Geometry: final body of the model. Coordinates: model frame, mm. A direction names the side the tool comes from. Give positions to 0.01 mm unless a question says otherwise; leave off trailing zeros. Order: outer loops, then holes, each group sorted by start corner. A loop starts at its lowest first (then second) coordinate and runs counter-clockwise, first axis right, second up. Notation, with made-up numbers: (52, 30.5) -> (70, 30.5) arc R6 cw to (70, 37.5) -> close; hole circle Ø8 at (57.5, 86). An arc over 180 degrees is marked (long way). One line per question, with ' | ' between items. Start each with the question number.
(1) Section D-D (x = 67.5). Return loops of the section in (y, z), then the cut area to 3 significant figures.
(2) Mould query, pull axis Y, two halves, no side actions, for faces 5 (the face through (45.44, 40.45, -2.54)), 6 (the face through (-3, 1, -2)), 7 (the face through (2, 3.05, -2)), 8 (the face through (35, 124, -2)). Classes: +Y half, -Y half, draft (parallel to the pull), parting line (faces both ways), or undercut.
(3) Ray query, L1, parallel to Y at x = 28, z = -59.5; L2, parallel to Y at x = 45, z = -3.2; L3, parallel to Z at x = 51, y = 67. Return the intervals inside material, ascending.
(4) First-contact query: pin 1 Ø12 at (y, z) = (80, -24) entering from -X; pin 2 Ø5.5 at (y, z) = (116.5, -3) entering from -X; pin 3 Ø4.5 at (x, z) = (-2, -3.5) entering from -Y. Flat tips, straight axial feed; report the tip coordinate or a pass-through.
(5) Set-up query: faces 1 (the face through (18, 149, -28)), 2 (the face through (-3, -1, -2)), 3 (the face through (50, 75.95, -32)), 4 (the face through (7, -3.05, -2)). Return all of +Z, -Z, +X, -X, +Y, -Y with unobstructed straight access to the full face (end or side cutting, diameter ignored); none if empty.
(6) Section C-C (y = 113). Return loops of the section in (x, z).
(7) Section A-A (z = -45). Return loops of the section in (x, y).
(8) Section B-B (x = 17.5). Return loops of the section in (y, z).
```python
from build123d import *

# Parameters (mm, degrees)
BOSS_EXTRUDE1_DEPTH = 5
BOSS_EXTRUDE2_DEPTH = 80
SKETCH4_W           = 4
SKETCH4_H           = 2
CUT_EXTRUDE1_DEPTH  = 73.715728753
SKETCH5_W           = 67.715728753
SKETCH5_H           = 50
CUT_EXTRUDE2_DEPTH  = 81
CUT_EXTRUDE3_DEPTH  = 65
SKETCH7_W           = 80
SKETCH7_H           = 5
BOSS_EXTRUDE3_DEPTH = 10.5
BOSS_EXTRUDE4_DEPTH = 80
FILLET1_R           = 2
FILLET2_R           = 10
CUT_EXTRUDE4_DEPTH  = 170.5
FILLET3_R           = 10
SKETCH10_R          = 3.4
CUT_EXTRUDE5_DEPTH  = 6


with BuildPart() as part:
    # Sketch2 → Boss-Extrude1 (new body)
    with BuildSketch(Plane.XY):
        Polygon((-5.152414984, 3.618325464), (-5.152414984, -3.618325464), (-1.641080211, -6.95), (-1, -6.95), (-1, -3.05), (95, -3.05), (95, 155.95), (5, 155.95), (5, 3.05), (-1, 3.05), (-1, 6.95), (-1.641080211, 6.95), align=None)
    extrude(amount=-BOSS_EXTRUDE1_DEPTH)

    # Sketch3 → Boss-Extrude2 (add)
    with BuildSketch(Plane(origin=(0, 155.95, 0), x_dir=(1, 0, 0), z_dir=(0, 1, 0))):
        with BuildLine():
            ThreePointArc((85, 72.715728753), (50, 56), (15, 72.715728753))
            Line((15, 72.715728753), (15, 5))
            Line((15, 5), (85, 5))
            Line((85, 5), (85, 72.715728753))
        make_face()
    extrude(amount=-BOSS_EXTRUDE2_DEPTH)

    # Sketch4 → Cut-Extrude1 (cut, through all)
    with BuildSketch(Plane.XY):
        with Locations((-3.152414984, 0)):
            Rectangle(SKETCH4_W, SKETCH4_H)
    extrude(amount=-CUT_EXTRUDE1_DEPTH, mode=Mode.SUBTRACT)

    # Sketch5 → Cut-Extrude2 (cut, through all)
    with BuildSketch(Plane.ZY.offset(-15)):
        with Locations((-38.857864377, 115.95)):
            Rectangle(SKETCH5_W, SKETCH5_H)
    extrude(amount=-CUT_EXTRUDE2_DEPTH, mode=Mode.SUBTRACT)

    # Sketch6 → Cut-Extrude3 (cut)
    with BuildSketch(Plane(origin=(0, 155.95, 0), x_dir=(1, 0, 0), z_dir=(0, 1, 0))):
        Polygon((35, 0), (35, 5), (20, 28), (15, 28), (15, 5), (5, 5), (5, 0), align=None)
    extrude(amount=-CUT_EXTRUDE3_DEPTH, mode=Mode.SUBTRACT)

    # Sketch7 → Boss-Extrude3 (add)
    with BuildSketch(Plane.XZ.offset(3.05)):
        with Locations((55, -2.5)):
            Rectangle(SKETCH7_W, SKETCH7_H)
    extrude(amount=BOSS_EXTRUDE3_DEPTH)

    # Sketch8 → Boss-Extrude4 (add)
    with BuildSketch(Plane.ZY.offset(-15)):
        Polygon((-5, -3.05), (-25, -13.55), (-5, -13.55), align=None)
    extrude(amount=-BOSS_EXTRUDE4_DEPTH)

    # Fillet1
    fillet1_edges = [part.edges().sort_by_distance(p)[0] for p in [
        (55, -13.55, -25),
    ]]
    fillet(fillet1_edges, radius=FILLET1_R)

    # Fillet2
    fillet2_edges = [part.edges().sort_by_distance(p)[0] for p in [
        (5, 90.95, -2.5),
    ]]
    fillet(fillet2_edges, radius=FILLET2_R)

    # Sketch9 → Cut-Extrude4 (cut, through all)
    with BuildSketch(Plane(origin=(0, 155.95, 0), x_dir=(1, 0, 0), z_dir=(0, 1, 0))):
        Polygon((85, 5), (85, 0), (95, 0), (95, 72.715728753), (85, 72.715728753), align=None)
    extrude(amount=-CUT_EXTRUDE4_DEPTH, mode=Mode.SUBTRACT)

    # Fillet3
    fillet3_edges = [part.edges().sort_by_distance(p)[0] for p in [
        (85, 83.45, -72.715728753),
        (85, 148.45, -72.715728753),
    ]]
    fillet(fillet3_edges, radius=FILLET3_R)

    # Sketch10 → Cut-Extrude5 (cut, through all)
    with BuildSketch(Plane(origin=(0, 0, -5), x_dir=(-1, 0, 0), z_dir=(0, 0, -1))):
        with Locations((-45, 37.07686976)):
            Circle(SKETCH10_R)
    extrude(amount=-CUT_EXTRUDE5_DEPTH, mode=Mode.SUBTRACT)


solid = part.part
```
Response:
1) outline: (-13.55, -16.89) arc R2 ccw to (-9.78, -17.82) -> (-3.05, -5) -> (75.95, -5) -> (75.95, -59.54) -> (90.95, -59.54) -> (90.95, -5) -> (140.95, -5) -> (140.95, -59.54) -> (155.95, -59.54) -> (155.95, 0) -> (-13.55, 0) -> close | area: 2,580 mm^2
2) face 5: undercut | face 6: undercut | face 7: +Y half | face 8: draft
3) L1: y = 75.95 to 90.95, 140.95 to 155.95 | L2: y = -13.55 to 33.68, 40.48 to 155.95 | L3: z = -5 to 0
4) pin 1: stops at x = 15 | pin 2: stops at x = 35 | pin 3: stops at y = -6.95
5) face 1: +Z, -X, +Y | face 2: +Z, -Z, -X | face 3: -Z, +X, -X | face 4: +Z, -Z, -Y
6) outline: (35, -5) -> (85, -5) -> (85, 0) -> (35, 0) -> close
7) outline: (15, 75.95) -> (85, 75.95) -> (85, 90.95) -> (15, 90.95) -> close; (15, 140.95) -> (85, 140.95) -> (85, 155.95) -> (15, 155.95) -> close
8) outline: (-13.55, -16.89) arc R2 ccw to (-9.78, -17.82) -> (-3.05, -5) -> (75.95, -5) -> (75.95, -69.88) -> (90.95, -69.88) -> (90.95, 0) -> (-13.55, 0) -> close; (140.95, -69.88) -> (155.95, -69.88) -> (155.95, -28) -> (140.95, -28) -> close
